Could you check a few things on this drawing? It's one solid part, dimensions in mm from its lowest x, y, z. A direction names the side the tool comes from. Round coordinates to 2 decimals unless told otherwise and drop trailing zeros. Loops run counter-clockwise (first coordinate to the right, second up) from the corner with the lowest first, then second, coordinate; pieces in that order, holes last. Notation, with made-up numbers: M 26,23.5 L 40,23.5 A17 ccw 40,33.5 Z; hole C 23,64.5 d2. An arc over 180 degrees is marked long. Return JSON: item names as keys, results as strings.
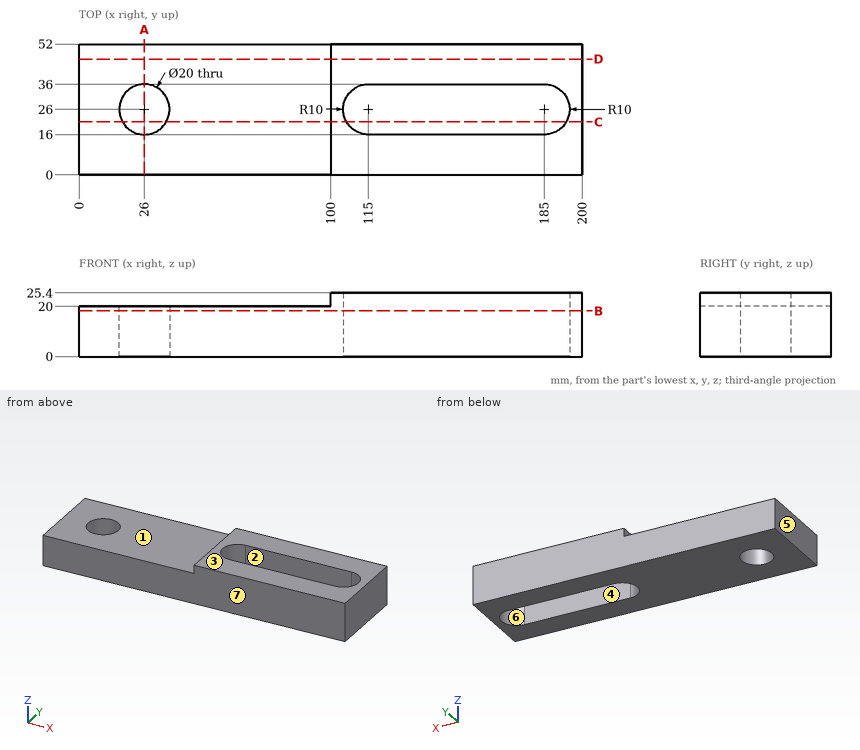
Q1. Thinking about a two-plate mould opening in X: for the marked faces 4, 5, 6 and 7, which applies, pulls with the +X half, pulls with the -X half, needs draft (parallel to the pull), parting line crosses it, or undercut?
Results:
{"face 4": "undercut", "face 5": "pulls with the -X half", "face 6": "undercut", "face 7": "needs draft"}
Q2. I'm going to push flat-ended pins straight in: pin 1 Ø5 at (y, z) = (14, 10.5) entering from -X; pin 2 Ø23 at (x, y) = (26, 26) entering from +Z. Where does each tip first touch, or does it pass through?
Results:
{"pin 1": "stops at x = 0", "pin 2": "stops at z = 20"}
Q3. Suppose I cut it at B-B, the plane z = 18.25. Please give me the cut outline in (x, y).
Results:
{"outline": "M 0,0 L 200,0 L 200,52 L 0,52 Z; hole C 26,26 d20; hole M 114.98,36 A10 ccw 115,16 L 185,16 A10 ccw 184.99,36 Z"}
Q4. On a 3-axis mill with a long thin cutter (end or side, diameter ignored), from which of +Z, -Z, +X, -X, +Y, -Y can I reach the whole of each face in a straight line? I mean the marked faces 1, 2 and 3. Say none if no direction works.
Results:
{"face 1": "+Z, -X, +Y, -Y", "face 2": "+Z, -Z", "face 3": "+Z, +X, -X, +Y, -Y"}
Q5. Suppose I cut it at A-A, the plane x = 26. Please give me the cut outline in (y, z), plus the area to 3 significant figures.
Results:
{"outline": "M 0,0 L 16,0 L 16,20 L 0,20 Z; M 36,0 L 52,0 L 52,20 L 36,20 Z", "area": "640 mm2"}
Q6. If I drill on line 1 along Y through (x, z) = (26, 9.5); line 2 along X through (y, z) = (33, 11.25); line 3 along X through (y, z) = (21, 3.5), over which ranges is the centre line in solid material (lowest first)?
Results:
{"line 1": "y = 0 to 16, 36 to 52", "line 2": "x = 0 to 18.86, 33.14 to 107.86, 192.14 to 200", "line 3": "x = 0 to 17.34, 34.66 to 106.34, 193.66 to 200"}
Q7. Suppose I cut it at C-C, the plane y = 21. Please give me the cut outline in (x, z).
Results:
{"outline": "M 0,0 L 17.34,0 L 17.34,20 L 0,20 Z; M 34.66,0 L 106.34,0 L 106.34,25.4 L 100,25.4 L 100,20 L 34.66,20 Z; M 193.66,0 L 200,0 L 200,25.4 L 193.66,25.4 Z"}
Q8. Suppose I cut it at D-D, the plane y = 46. Please give me the cut outline in (x, z).
Results:
{"outline": "M 0,0 L 200,0 L 200,25.4 L 100,25.4 L 100,20 L 0,20 Z"}
